Source: CAD feature listing. Evaluate the final solid. Frame: model axes, mm. A direction names the side the tool comes from. Give positions to 0.01 mm unless a question says otherwise; leave off trailing zeros. Order: outer loops, then holes, each group sorted by start corner. A loop starts at its lowest first (then second) coordinate and runs counter-clockwise, first axis right, second up.
from build123d import *

# Parameters (mm, degrees)
SKETCH_1_W               = 25.9
SKETCH_1_H               = 8.5
EXTRUDE_1_DEPTH          = 2.5
SKETCH_1_5_W             = 23.6
SKETCH_1_5_H             = 1.5
EXTRUDE_2_DEPTH          = 2.5
SKETCH_2_W               = 23.6
SKETCH_2_H               = 1.5
EXTRUDE_3_DEPTH          = 3.1
SKETCH_3_W               = 1.8
SKETCH_3_H               = 5.6
CUT_EXTRUDE_1_DEPTH      = 1.5
CUT_EXTRUDE_2_DEPTH      = 2
CUT_EXTRUDE_2_DEPTH_BACK = 10
SKETCH_4_W               = 8.769979371
SKETCH_4_H               = 7.729949766


with BuildPart() as part:
    # 草图1 → 凸台-拉伸1 (new body)
    with BuildSketch(Plane.XY):
        with Locations((7.382170543, 0.04770021)):
            Rectangle(SKETCH_1_W, SKETCH_1_H)
    extrude(amount=EXTRUDE_1_DEPTH)

    # 草图1<5> → 凸台-拉伸2 (add)
    with BuildSketch(Plane.XY):
        with Locations((7.382170543, 5.04770021)):
            Rectangle(SKETCH_1_5_W, SKETCH_1_5_H)
    extrude(amount=EXTRUDE_2_DEPTH)

    # 草图2 → 凸台-拉伸3 (add)
    with BuildSketch(Plane.XY.offset(2.5)):
        with Locations((7.382170543, 5.04770021)):
            Rectangle(SKETCH_2_W, SKETCH_2_H)
    extrude(amount=EXTRUDE_3_DEPTH)

    # 草图3 → 切除-拉伸1 (cut)
    with BuildSketch(Plane(origin=(0, 5.79770021, 0), x_dir=(1, 0, 0), z_dir=(0, 1, 0))):
        with Locations((17.542170543, -2.8)):
            Rectangle(SKETCH_3_W, SKETCH_3_H)
        with Locations((15.002170543, -2.8)):
            Rectangle(SKETCH_3_W, SKETCH_3_H)
        with Locations((12.462170543, -2.8)):
            Rectangle(SKETCH_3_W, SKETCH_3_H)
        with Locations((9.922170543, -2.8)):
            Rectangle(SKETCH_3_W, SKETCH_3_H)
        with Locations((7.382170543, -2.8)):
            Rectangle(SKETCH_3_W, SKETCH_3_H)
        with Locations((4.842170543, -2.8)):
            Rectangle(SKETCH_3_W, SKETCH_3_H)
        with Locations((2.302170543, -2.8)):
            Rectangle(SKETCH_3_W, SKETCH_3_H)
        with Locations((-0.237829457, -2.8)):
            Rectangle(SKETCH_3_W, SKETCH_3_H)
        with Locations((-2.777829457, -2.8)):
            Rectangle(SKETCH_3_W, SKETCH_3_H)
    extrude(amount=-CUT_EXTRUDE_1_DEPTH, mode=Mode.SUBTRACT)

    # 草图4 → 切除-拉伸2 (cut, two sides: drawn at the far end of the back side and taken through both)
    with BuildSketch(Plane(origin=(0, 4.29770021, 0), x_dir=(1, 0, 0), z_dir=(0, 1, 0)).offset(-CUT_EXTRUDE_2_DEPTH_BACK)):
        with Locations((16.847160229, -2.378366376)):
            Rectangle(SKETCH_4_W, SKETCH_4_H)
    extrude(amount=CUT_EXTRUDE_2_DEPTH + CUT_EXTRUDE_2_DEPTH_BACK, mode=Mode.SUBTRACT)


solid = part.part
1) Pull-direction query (X, two-part tool) for faces 1 (the face through (-4.418, 5, 3)), 2 (the face through (-5, 4.298, 1)), 3 (the face through (0.662, 5, 3)); classes: +X half, -X half, draft (parallel to the pull), parting line (faces both ways), or undercut.
Checks:
face 1: -X half
face 2: draft
face 3: undercut
2) First-contact query: pin 1 Ø0.8 at (x, z) = (1, 3.5) entering from -Y; pin 2 Ø0.8 at (y, z) = (5.5, 2) entering from -X; pin 3 Ø1.2 at (y, z) = (5, 1.5) entering from +X. Flat tips, straight axial feed; report the tip coordinate or a pass-through.
Checks:
pin 1: stops at y = 4.3
pin 2: stops at x = -4.42
pin 3: stops at x = 11.56
3) Section query D-D on y = -1. Output: boundary loops of the cut face in (x, z), and give its area (3 significant figures).
Checks:
outline: (-5.57, 0) - (12.46, 0) - (12.46, 2.5) - (-5.57, 2.5) - close
area: 45.1 mm2
4) Ray query, L1, parallel to Z at x = 6.25, y = -3.5; L2, parallel to Y at x = 4.75, z = 2.2; L3, parallel to Y at x = 6.25, z = 5.05. Return the intervals inside material, ascending.
Checks:
L1: z = 0 to 2.5
L2: y = -4.2 to 4.3
L3: y = 4.3 to 5.8
5) Reachability of faces 4 (the face through (-5.568, 0, 1)), 5 (the face through (12, 4.298, 1)), 6 (the face through (1.402, 5, 3)) from +Z, -Z, +X, -X, +Y, -Y: full face, straight path, thin tool, end or side. Return the list, or none.
Checks:
face 4: +Z, -Z, -X, +Y, -Y
face 5: +Z, -Z, +X, +Y
face 6: +Z, -Z, +Y
6) Section query A-A on y = 4.75. Output: boundary loops of the cut face in (x, z), and give its area (3 significant figures).
Checks:
outline: (-4.42, 0) - (-3.68, 0) - (-3.68, 5.6) - (-4.42, 5.6) - close; (-1.88, 0) - (-1.14, 0) - (-1.14, 5.6) - (-1.88, 5.6) - close; (0.66, 0) - (1.4, 0) - (1.4, 5.6) - (0.66, 5.6) - close; (3.2, 0) - (3.94, 0) - (3.94, 5.6) - (3.2, 5.6) - close; (5.74, 0) - (6.48, 0) - (6.48, 5.6) - (5.74, 5.6) - close; (8.28, 0) - (9.02, 0) - (9.02, 5.6) - (8.28, 5.6) - close; (10.82, 0) - (11.56, 0) - (11.56, 5.6) - (10.82, 5.6) - close
area: 29.0 mm2
7) Section query B-B on z = 4.7. Output: boundary loops of the cut face in (x, y), and give its area (3 significant figures).
Checks:
outline: (-4.42, 4.3) - (-3.68, 4.3) - (-3.68, 5.8) - (-4.42, 5.8) - close; (-1.88, 4.3) - (-1.14, 4.3) - (-1.14, 5.8) - (-1.88, 5.8) - close; (0.66, 4.3) - (1.4, 4.3) - (1.4, 5.8) - (0.66, 5.8) - close; (3.2, 4.3) - (3.94, 4.3) - (3.94, 5.8) - (3.2, 5.8) - close; (5.74, 4.3) - (6.48, 4.3) - (6.48, 5.8) - (5.74, 5.8) - close; (8.28, 4.3) - (9.02, 4.3) - (9.02, 5.8) - (8.28, 5.8) - close; (10.82, 4.3) - (11.56, 4.3) - (11.56, 5.8) - (10.82, 5.8) - close
area: 7.77 mm2
